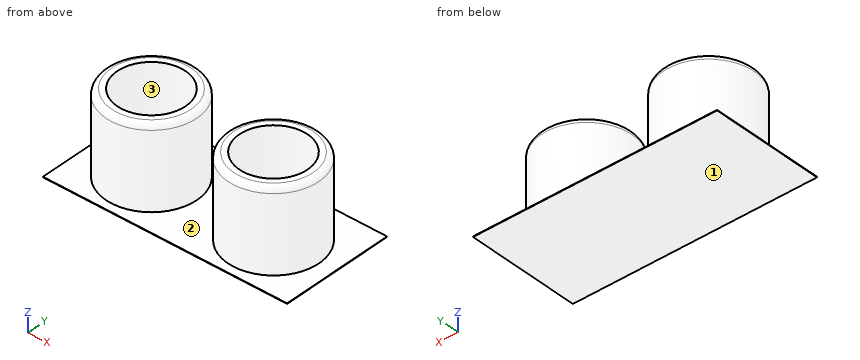
from build123d import *

# Parameters (mm, degrees)
SKETCH1_W           = 43
SKETCH1_H           = 20
BOSS_EXTRUDE1_DEPTH = 0.1
SKETCH3_R           = 8
BOSS_EXTRUDE2_DEPTH = 14.4
FILLET1_R           = 1
SKETCH5_R           = 6
CUT_EXTRUDE1_DEPTH  = 10


with BuildPart() as part:
    # Sketch1 → Boss-Extrude1 (new body)
    with BuildSketch(Plane.XY):
        with Locations((0, 0.508181818)):
            Rectangle(SKETCH1_W, SKETCH1_H)
    extrude(amount=BOSS_EXTRUDE1_DEPTH)

    # Sketch3 → Boss-Extrude2 (add)
    with BuildSketch(Plane.XY.offset(0.1)):
        with Locations((-10.75, 0)):
            Circle(SKETCH3_R)
        with Locations(Location((10.75, 0, 0), (0, 0, 180))):
            Circle(SKETCH3_R)
    extrude(amount=BOSS_EXTRUDE2_DEPTH)

    # Fillet1
    fillet1_edges = [part.edges().sort_by_distance(p)[0] for p in [
        (-18.75, 0, 14.5),
        (18.75, 0, 14.5),
    ]]
    fillet(fillet1_edges, radius=FILLET1_R)

    # Sketch5 → Cut-Extrude1 (cut)
    with BuildSketch(Plane.XY.offset(14.5)):
        with Locations((-10.75, 0)):
            Circle(SKETCH5_R)
        with Locations(Location((10.75, 0, 0), (0, 0, 180))):
            Circle(SKETCH5_R)
    extrude(amount=-CUT_EXTRUDE1_DEPTH, mode=Mode.SUBTRACT)


solid = part.part
Geometry check sheet. Reference: the model listing, model coordinates, mm. Face numbers are marked on the shaded views. Round coordinates to 2 decimals unless told otherwise and drop trailing zeros. Order: outer loops, then holes, each group sorted by start corner. A loop starts at its lowest first (then second) coordinate and runs counter-clockwise, first axis right, second up. Notation, with made-up numbers: M 24,38.25 L 81,38.25 A17 ccw 81,65.25 Z; hole C 0.25,-25 d3. An arc over 180 degrees is marked long. Write each question's results on one line, items separated by ' | '. Start each with the question number.
1. Draft check along X on the marked faces 1, 2 and 3. Enter one of: pulls with the +X half, pulls with the -X half, needs draft (parallel to the pull), parting line crosses it, or undercut.
2. Material ranges on L1, parallel to Y at x = 10.75, z = 12; L2, parallel to X at y = 2.25, z = 13.25; L3, parallel to X at y = -5, z = 6.5 (3 decimals), recorded low to high. Write a range as from..to.
3. Go/stop test with flat-tipped pins: P1, Ø3, axis at y = 4, z = 5, coming from the -X side; P2, Ø7, axis at x = -10.75, y = 0, coming from the +Z side; P3, Ø4, axis at x = -14.5, z = 11, coming from the +Y side. Record where each tip stops, or that it passes through.
4. Cross-section at A-A on x = -10.75. Record the boundary of the cut face in (y, z), plus the area to 3 significant figures.
5. Cross-section at B-B on y = 0. Record the boundary of the cut face in (x, z).
6. Cross-section at C-C on z = 3.25. Record the boundary of the cut face in (x, y), plus the area to 3 significant figures.
7. Cross-section at D-D on z = 9.5. Record the boundary of the cut face in (x, y).
Resolved:
1) face 1: needs draft | face 2: undercut | face 3: undercut
2) L1: -8..-6, 6..8 | L2: -18.43..-16.31, -5.19..-3.07, 3.07..5.19, 16.31..18.43 | L3: -16.995..-14.067, -7.433..-4.505, 4.505..7.433, 14.067..16.995
3) P1: x = -18.35 | P2: z = 4.5 | P3: y = 7.81
4) outline: M -9.49,0 L 10.51,0 L 10.51,0.1 L 8,0.1 L 8,13.5 A1 ccw 7,14.5 L 6,14.5 L 6,4.5 L -6,4.5 L -6,14.5 L -7,14.5 A1 ccw -8,13.5 L -8,0.1 L -9.49,0.1 Z | area: 112 mm2
5) outline: M -21.5,0 L 21.5,0 L 21.5,0.1 L 18.75,0.1 L 18.75,13.5 A1 ccw 17.75,14.5 L 16.75,14.5 L 16.75,4.5 L 4.75,4.5 L 4.75,14.5 L 3.75,14.5 A1 ccw 2.75,13.5 L 2.75,0.1 L -2.75,0.1 L -2.75,13.5 A1 ccw -3.75,14.5 L -4.75,14.5 L -4.75,4.5 L -16.75,4.5 L -16.75,14.5 L -17.75,14.5 A1 ccw -18.75,13.5 L -18.75,0.1 L -21.5,0.1 Z
6) outline: C -10.75,0 d16; C 10.75,0 d16 | area: 402 mm2
7) outline: C -10.75,0 d16; C 10.75,0 d16; hole C -10.75,0 d12; hole C 10.75,0 d12
